The model under review builds one solid part; all positions refer to its coordinate system, in mm. A direction names the side the tool comes from. Coordinates: 2 decimals unless noted, no trailing zeros. Write each loop counter-clockwise with the first axis right and the second up, starting at its lowest first coordinate (ties: lowest second). Pieces come first, ordered by that corner, then holes. Notation, with made-up numbers: (-10.75, 47) - (-1.75, 47) arc R24 cw to (-1.75, 58) - close; hole circle Ø9 at (69, -18). An arc over 180 degrees is marked (long way). Put each result on its own line as item: value.
from build123d import *

# Parameters (mm, degrees)
F0_W     = 345.44
F0_H     = 143.9926
F0_R     = 6.7437
F0_R_2   = 5.207
F0_R_3   = 6.75
F1_DEPTH = 18.9992
F2_W     = 6.35
F2_H     = 25.4
F3_DEPTH = 345.441
F4_W     = 34.925
F4_H     = 37.58184
F5_DEPTH = 6.35


with BuildPart() as f1:
    # F0 (on Front) → F1 (new body)
    with BuildSketch(Plane.XZ):
        Rectangle(F0_W, F0_H)
        with Locations((-87.884, -59.9948)):
            Circle(F0_R, mode=Mode.SUBTRACT)
        with Locations((-115.57, -47.11446)):
            Circle(F0_R_2, mode=Mode.SUBTRACT)
        with Locations((-64.77, -47.11446)):
            Circle(F0_R_2, mode=Mode.SUBTRACT)
        with Locations((-13.97, -47.11446)):
            Circle(F0_R_2, mode=Mode.SUBTRACT)
        with Locations((153.67, -59.9948)):
            Circle(F0_R_3, mode=Mode.SUBTRACT)
        with Locations((-87.884, 59.9948)):
            Circle(F0_R, mode=Mode.SUBTRACT)
        with Locations((153.67, 59.9948)):
            Circle(F0_R, mode=Mode.SUBTRACT)
    extrude(amount=F1_DEPTH)

    # F2 (on face) → F3 (cut, through all)
    with BuildSketch(Plane(origin=(-172.72, 0, 0), x_dir=(0, -1, 0), z_dir=(-1, 0, 0))):
        with Locations((3.175, -47.11446)):
            Rectangle(F2_W, F2_H)
    extrude(amount=-F3_DEPTH, mode=Mode.SUBTRACT)

    # F4 (on face) → F5 (cut, through all)
    with BuildSketch(Plane(origin=(0, 0, 0), x_dir=(-1, 0, 0), z_dir=(0, 1, 0))):
        with Locations((-155.2575, -53.20538)):
            Rectangle(F4_W, F4_H)
        with Locations((155.2575, -53.20538)):
            Rectangle(F4_W, F4_H)
    extrude(amount=-F5_DEPTH, mode=Mode.SUBTRACT)


solid = f1.part
1. Consider section C-C on y = -14.5. State the section outline as (x, z) points, plus the area to 3 significant figures.
Determined:
outline: (-172.72, -72) - (172.72, -72) - (172.72, 72) - (-172.72, 72) - close; hole circle Ø10.41 at (-115.57, -47.11); hole circle Ø13.49 at (-87.88, -59.99); hole circle Ø13.49 at (-87.88, 59.99); hole circle Ø10.41 at (-64.77, -47.11); hole circle Ø10.41 at (-13.97, -47.11); hole circle Ø13.5 at (153.67, -59.99); hole circle Ø13.49 at (153.67, 59.99)
area: 48,900 mm^2
2. The part is to be moulded in two halves that separate along Z. For faces 4 (the cylindrical face through (-88.76, -9.37, 66.68)), 5 (the flat face through (-2, -9, 71.996)), 6 (the flat face through (-2, -9, -71.996)), 7 (the flat face through (-137.795, -3, -66)), say which applies: +Z half, -Z half, draft (parallel to the pull), parting line (faces both ways), or undercut.
Determined:
face 4: undercut
face 5: +Z half
face 6: -Z half
face 7: draft
3. Consider section A-A on x = -115.57. State the section outline as (y, z) points.
Determined:
outline: (-19, -72) - (0, -72) - (0, -59.81) - (-6.35, -59.81) - (-6.35, -52.32) - (-19, -52.32) - close; (-19, -41.91) - (-6.35, -41.91) - (-6.35, -34.41) - (0, -34.41) - (0, 72) - (-19, 72) - close
4. Machinability: for faces 1 (the cylindrical face through (160.102, -9.367, 62.02)), 2 (the flat face through (137.795, -3, -66)), 3 (the flat face through (-117, -3, -59.814)), which of the approach directions +Z, -Z, +X, -X, +Y, -Y give a long, thin tool a straight path to every point of the face, cutting with its end or side? Answer none if there is none.
Determined:
face 1: +Y, -Y
face 2: -Z, +X, +Y
face 3: +X, -X, +Y
5. For pin 1 Ø15.5 at (x, z) = (-87.88, -59.99) entering from -Y; pin 2 Ø3 at (y, z) = (-2, -68) entering from +X (3 decimals); pin 3 Ø3 at (y, z) = (-3.5, -63.5) entering from -X (3 decimals), all flat-tipped, find the tip position at first contact; note any pin that passes through.
Determined:
pin 1: stops at y = -19
pin 2: stops at x = 137.795
pin 3: stops at x = -137.795
6. To check wall thickness, follow probe 1 along Z at (x, y) = (153.67, -10.25); probe 2 along Z at (x, y) = (-87, -17.75); probe 3 along Z at (x, y) = (-17.5, -6). State the ranges of each line that lie inside material, in increasing order.
Determined:
probe 1: z = -72 to -66.74, -53.24 to 53.25, 66.74 to 72
probe 2: z = -72 to -66.68, -53.31 to 53.31, 66.68 to 72
probe 3: z = -72 to -59.81, -34.41 to 72
7. Consider section B-B on x = 153.67. State the section outline as (y, z) points, plus the area to 3 significant figures.
Determined:
outline: (-19, -72) - (-6.35, -72) - (-6.35, -66.74) - (-19, -66.74) - close; (-19, -53.24) - (-6.35, -53.24) - (-6.35, -34.41) - (0, -34.41) - (0, 53.25) - (-19, 53.25) - close; (-19, 66.74) - (0, 66.74) - (0, 72) - (-19, 72) - close
area: 2,070 mm^2
